from build123d import *

# Parameters (mm, degrees)
SKETCH1_W           = 39
SKETCH1_H           = 11.5
BOSS_EXTRUDE1_DEPTH = 17
SKETCH2_W           = 5
SKETCH2_H           = 2.5
SKETCH2_H_2         = 2
BOSS_EXTRUDE2_DEPTH = 9
FILLET3_R           = 1
FILLET4_R           = 1
FILLET5_R           = 1
FILLET6_R           = 1
CHAMFER1_SIZE       = 10
CHAMFER2_SIZE       = 10
SKETCH4_W           = 4.09
SKETCH4_H           = 3.02
CUT_EXTRUDE1_DEPTH  = 2
SKETCH5_W           = 45.21307777
SKETCH5_H           = 21.662699148
CUT_EXTRUDE2_DEPTH  = 6
FILLET7_R           = 5
FILLET8_R           = 5


with BuildPart() as part:
    # Sketch1 → Boss-Extrude1 (new body)
    with BuildSketch(Plane.XY):
        with Locations((19.5, -5.75)):
            Rectangle(SKETCH1_W, SKETCH1_H)
    extrude(amount=BOSS_EXTRUDE1_DEPTH)

    # Sketch2 → Boss-Extrude2 (add)
    with BuildSketch(Plane(origin=(0, 0, 0), x_dir=(-1, 0, 0), z_dir=(0, 0, -1))):
        with Locations((-2.5, -10.25)):
            Rectangle(SKETCH2_W, SKETCH2_H)
        with Locations((-2.5, -1)):
            Rectangle(SKETCH2_W, SKETCH2_H_2)
        with Locations((-36.5, -10.25)):
            Rectangle(SKETCH2_W, SKETCH2_H)
        with Locations((-36.5, -1)):
            Rectangle(SKETCH2_W, SKETCH2_H_2)
    extrude(amount=BOSS_EXTRUDE2_DEPTH)

    # Fillet3
    fillet3_edges = [part.edges().sort_by_distance(p)[0] for p in [
        (34, -1, 0),
    ]]
    fillet(fillet3_edges, radius=FILLET3_R)

    # Fillet4
    fillet4_edges = [part.edges().sort_by_distance(p)[0] for p in [
        (5, -1, 0),
    ]]
    fillet(fillet4_edges, radius=FILLET4_R)

    # Fillet5
    fillet5_edges = [part.edges().sort_by_distance(p)[0] for p in [
        (34, -10.25, 0),
    ]]
    fillet(fillet5_edges, radius=FILLET5_R)

    # Fillet6
    fillet6_edges = [part.edges().sort_by_distance(p)[0] for p in [
        (5, -10.25, 0),
    ]]
    fillet(fillet6_edges, radius=FILLET6_R)

    # Chamfer1
    chamfer1_edges = [part.edges().sort_by_distance(p)[0] for p in [
        (39, -5.75, 17),
    ]]
    chamfer(chamfer1_edges, length=CHAMFER1_SIZE)

    # Chamfer2
    chamfer2_edges = [part.edges().sort_by_distance(p)[0] for p in [
        (0, -5.75, 17),
    ]]
    chamfer(chamfer2_edges, length=CHAMFER2_SIZE)

    # Sketch4 → Cut-Extrude1 (cut)
    with BuildSketch(Plane(origin=(0, 0, 0), x_dir=(1, 0, 0), z_dir=(0, 1, 0))):
        with Locations((26.955, -15.49)):
            Rectangle(SKETCH4_W, SKETCH4_H)
        with Locations((12.045, -15.49)):
            Rectangle(SKETCH4_W, SKETCH4_H)
    extrude(amount=-CUT_EXTRUDE1_DEPTH, mode=Mode.SUBTRACT)

    # Sketch5 → Cut-Extrude2 (cut)
    with BuildSketch(Plane.XZ.offset(11.5)):
        with Locations((22.606538885, 14.331349574)):
            Rectangle(SKETCH5_W, SKETCH5_H)
    extrude(amount=-CUT_EXTRUDE2_DEPTH, mode=Mode.SUBTRACT)

    # Fillet7
    fillet7_edges = [part.edges().sort_by_distance(p)[0] for p in [
        (0, -2.75, 7),
    ]]
    fillet(fillet7_edges, radius=FILLET7_R)

    # Fillet8
    fillet8_edges = [part.edges().sort_by_distance(p)[0] for p in [
        (39, -2.75, 7),
    ]]
    fillet(fillet8_edges, radius=FILLET8_R)


solid = part.part
Source: CAD feature listing. Evaluate the final solid. Frame: model axes, mm. A direction names the side the tool comes from. Round coordinates to 2 decimals unless told otherwise and drop trailing zeros. Loops run counter-clockwise (first coordinate to the right, second up) from the corner with the lowest first, then second, coordinate; pieces in that order, holes last. Notation, with made-up numbers: M 74.5,23.5 L 82.5,23.5 A22 cw 82.5,44.5 Z; hole C 21,-39.75 d4. An arc over 180 degrees is marked long. Return JSON: item names as keys, results as strings. Group by question number.
1. Section query C-C on y = -2.75. Output: boundary loops of the cut face in (x, z), and give its area (3 significant figures).
2. Material intervals for line 1 along X through (y, z) = (-9.5, -5); line 2 along Y through (x, z) = (37, -0.75); line 3 along Z through (x, y) = (17, -9.75), sorted ascending. Write a range as from..to.
3. Pin query (flat end, axial travel): pin 1 (6 mm diameter, centred on x = 4, y = -6, fed in from +Z); pin 2 (4 mm diameter, centred on y = -2, z = 14, fed in from -X); pin 3 (11 mm diameter, centred on x = 21, z = 10.5, fed in from -Y); pin 4 (3 mm diameter, centred on x = 35.5, z = -4, fed in from +Y). Return the tip coordinate at first contact, or that it passes through.
4. Reachability of faces 4 (the face through (12, -1, 13.98)), 5 (the face through (37, -9, -4)), 6 (the face through (33.715, -10.232, -0.301)) from +Z, -Z, +X, -X, +Y, -Y: full face, straight path, thin tool, end or side. Return the list, or none.
5. Section query B-B on z = -0.5. Output: boundary loops of the cut face in (x, y), and give its area (3 significant figures).
6. Mould query, pull axis X, two halves, no side actions, for faces 1 (the face through (19, -3, 17)), 2 (the face through (14.09, -1, 16)), 3 (the face through (33, -3, 13)). Classes: released by +X, released by -X, zero draft, split by the parting line, or undercut.
7. Section query A-A on x = 36. Output: boundary loops of the cut face in (y, z).
8. Section query D-D on x = 8. Output: boundary loops of the cut face in (y, z).
Checks:
{
 "1": {"outline": "M 0,0 L 39,0 L 39,4.93 A5 ccw 37.54,8.46 L 29,17 L 10,17 L 1.46,8.46 A5 ccw 0,4.93 Z", "area": "562 mm²"},
 "2": {"line 1": "x = 0..5, 34..39", "line 2": "y = -11.5..-9, -2..0", "line 3": "z = 0..3.5"},
 "3": {"pin 1": "stops at z = 13.96", "pin 2": "stops at x = 5", "pin 3": "stops at y = -5.5", "pin 4": "stops at y = 0"},
 "4": {"face 4": "+Z, +Y", "face 5": "-Z, +X, -X", "face 6": "-Z, +Y, -Y"},
 "5": {"outline": "M 0,-11.5 L 5.13,-11.5 L 5.13,-9 L 0,-9 Z; M 0,-2 L 5.13,-2 L 5.13,0 L 0,0 Z; M 33.87,-11.5 L 39,-11.5 L 39,-9 L 33.87,-9 Z; M 33.87,-2 L 39,-2 L 39,0 L 33.87,0 Z", "area": "46.2 mm²"},
 "6": {"face 1": "zero draft", "face 2": "undercut", "face 3": "released by +X"},
 "7": {"outline": "M -11.5,-9 L -9,-9 L -9,0 L -2,0 L -2,-9 L 0,-9 L 0,10 L -5.5,10 L -5.5,3.5 L -11.5,3.5 Z"},
 "8": {"outline": "M -11.5,0 L 0,0 L 0,15 L -5.5,15 L -5.5,3.5 L -11.5,3.5 Z"}
}
